Source: CAD feature listing. Evaluate the final solid. Frame: model axes, mm. Round coordinates to 2 decimals unless told otherwise and drop trailing zeros. Order: outer loops, then holes, each group sorted by start corner. A loop starts at its lowest first (then second) coordinate and runs counter-clockwise, first axis right, second up. Notation, with made-up numbers: (51, -4.5) -> (100, -4.5) arc R27 cw to (100, 16.5) -> close; hole circle Ø5 at (75.25, -8.75). An arc over 180 degrees is marked (long way). One line per item, written item: value. Start each with the question number.
1) Section B-B (x = 19). Return the cut outline in (y, z).
2) Section A-A (z = 0.3). Return the cut outline in (x, y), and give its area (3 significant figures).
3) Pin query (flat end, axial travel): P1, Ø3, axis at x = 5, y = 85, coming from the -Z side. Return the tip coordinate at first contact, or that it passes through.
4) Ray query, L1, parallel to Y at x = 86.5, z = 0.25; L2, parallel to X at y = 50, z = 0.35. Return the intervals inside material, ascending.
```python
from build123d import *

# Parameters (mm, degrees)
BOARD_DEPTH               = 0.41148
OTW_R_1_0_228_1_OUTLINE_R = 2.5
OTW_R_1_0_228_1_DEPTH     = 0.41148
OTW_R_1_0_228_2_OUTLINE_R = 2.5
OTW_R_1_0_228_2_DEPTH     = 0.41148
OTW_R_1_0_228_3_OUTLINE_R = 2.5
OTW_R_1_0_228_3_DEPTH     = 0.41148
OTW_R_1_0_228_4_OUTLINE_R = 2.5
OTW_R_1_0_228_4_DEPTH     = 0.41148


# Read off the part's stored shape, not the designer's step: Otwór #1 (0.228)1, Otwór #1 (0.228)2, Otwór #1 (0.228)3, Otwór #1 (0.228)4
with BuildPart() as part:
    # Szkic1 → Board (new body)
    with BuildSketch(Plane.XY):
        Polygon((90, 80), (85, 75), (85, 15), (90, 10), (90, 0), (80, 0), (75, 5), (15, 5), (10, 0), (0, 0), (0, 10), (5, 15), (5, 75), (0, 80), (0, 90), (10, 90), (15, 85), (75, 85), (80, 90), (90, 90), align=None)
    extrude(amount=BOARD_DEPTH)

    # Otwór #1 (0.228)1 outline → Otwór #1 (0.228)1 (cut)
    with BuildSketch(Plane.XY):
        with Locations((85, 85)):
            Circle(OTW_R_1_0_228_1_OUTLINE_R)
    extrude(amount=OTW_R_1_0_228_1_DEPTH, mode=Mode.SUBTRACT)

    # Otwór #1 (0.228)2 outline → Otwór #1 (0.228)2 (cut)
    with BuildSketch(Plane.XY):
        with Locations((5, 85)):
            Circle(OTW_R_1_0_228_2_OUTLINE_R)
    extrude(amount=OTW_R_1_0_228_2_DEPTH, mode=Mode.SUBTRACT)

    # Otwór #1 (0.228)3 outline → Otwór #1 (0.228)3 (cut)
    with BuildSketch(Plane.XY):
        with Locations((85, 5)):
            Circle(OTW_R_1_0_228_3_OUTLINE_R)
    extrude(amount=OTW_R_1_0_228_3_DEPTH, mode=Mode.SUBTRACT)

    # Otwór #1 (0.228)4 outline → Otwór #1 (0.228)4 (cut)
    with BuildSketch(Plane.XY):
        with Locations((5, 5)):
            Circle(OTW_R_1_0_228_4_OUTLINE_R)
    extrude(amount=OTW_R_1_0_228_4_DEPTH, mode=Mode.SUBTRACT)


solid = part.part
```
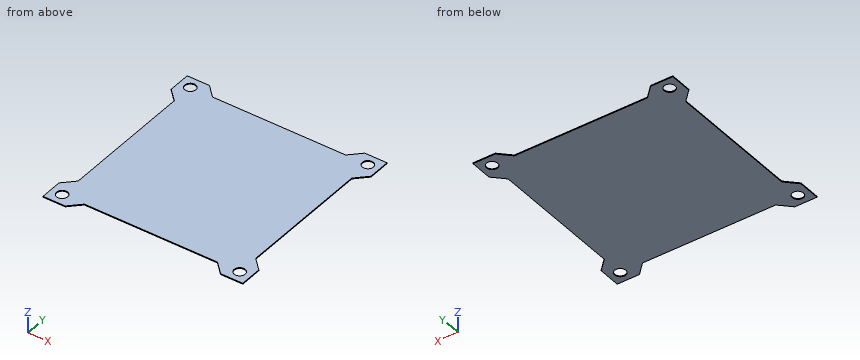
Findings:
1. outline: (5, 0) -> (85, 0) -> (85, 0.41) -> (5, 0.41) -> close
2. outline: (0, 0) -> (10, 0) -> (15, 5) -> (75, 5) -> (80, 0) -> (90, 0) -> (90, 10) -> (85, 15) -> (85, 75) -> (90, 80) -> (90, 90) -> (80, 90) -> (75, 85) -> (15, 85) -> (10, 90) -> (0, 90) -> (0, 80) -> (5, 75) -> (5, 15) -> (0, 10) -> close; hole circle Ø5 at (5, 5); hole circle Ø5 at (5, 85); hole circle Ø5 at (85, 5); hole circle Ø5 at (85, 85)
2. area: 6,720 mm2
3. P1: through
4. L1: 0 to 3, 7 to 13.5, 76.5 to 83, 87 to 90
4. L2: 5 to 85
